from build123d import *

# Parameters (mm, degrees)
F0_W     = 400
F0_H     = 500
F1_DEPTH = 750
F3_DEPTH = 20
F4_W     = 380
F4_H     = 480
F5_DEPTH = 618.889272


with BuildPart() as f1:
    # F0 (on Front) → F1 (new body)
    with BuildSketch(Plane.XZ):
        with Locations((200, 250)):
            Rectangle(F0_W, F0_H)
    extrude(amount=F1_DEPTH)

    # F2 (on face) → F3 (cut)
    with BuildSketch(Plane.XZ.offset(750)):
        Polygon((50, 70), (56, 70), (344, 430), (50, 430), align=None)
        Polygon((344, 430), (56, 70), (350, 70), (350, 430), align=None)
    extrude(amount=-F3_DEPTH, mode=Mode.SUBTRACT)

    # F4 (on face) → F5 (cut)
    with BuildSketch(Plane.XZ.offset(730)):
        with Locations((200, 250)):
            Rectangle(F4_W, F4_H)
    extrude(amount=-F5_DEPTH, mode=Mode.SUBTRACT)


solid = f1.part
Verification items for the finished model (mm, model axes). A direction names the side the tool comes from. Give positions to 0.01 mm unless a question says otherwise; leave off trailing zeros. Write each loop counter-clockwise with the first axis right and the second up, starting at its lowest first coordinate (ties: lowest second). Pieces come first, ordered by that corner, then holes. Notation, with made-up numbers: (83.25, 40) -> (101.25, 40) arc R16 ccw to (101.25, 69) -> close; hole circle Ø4 at (59.25, -18). An arc over 180 degrees is marked (long way). Use CSV: the item, a comma, the result in double quotes.
(1) Set-up check for faces 5 (the flat face through (350, -740, 247)), 6 (the flat face through (390, -425, 247)), 7 (the flat face through (400, -370, 247)): record each of +Z, -Z, +X, -X, +Y, -Y from which the full face is reachable in a straight line by a thin tool's end or side.
Derived:
face 5,"-Y"
face 6,"none"
face 7,"+Z, -Z, +X, +Y, -Y"
(2) Sectioned sample at A-A (x = 362). Record the cut outline in (y, z).
Derived:
outline,"(-750, 0) -> (0, 0) -> (0, 500) -> (-750, 500) -> close; hole (-730, 10) -> (-111.11, 10) -> (-111.11, 490) -> (-730, 490) -> close"
(3) Release check for a two-part mould opening along Y. For faces 1 (the flat face through (10, -425, 247)), 2 (the flat face through (197, 0, 254)), 3 (the flat face through (202, -740, 430)), 4 (the flat face through (375, -750, 254)) record: +Y half, -Y half, draft (parallel to the pull), parting line (faces both ways), or undercut.
Derived:
face 1,"undercut"
face 2,"+Y half"
face 3,"draft"
face 4,"-Y half"
(4) Material ranges on L1, parallel to Y at x = 20, z = 186; L2, parallel to Z at x = 285.5, y = -137.5; L3, parallel to X at y = -637.5, z = 77, recorded low to high.
Derived:
L1,"y = -750 to -730, -111.11 to 0"
L2,"z = 0 to 10, 490 to 500"
L3,"x = 0 to 10, 390 to 400"
(5) Sectioned sample at D-D (x = 148.5). Record the cut outline in (y, z).
Derived:
outline,"(-750, 0) -> (0, 0) -> (0, 500) -> (-750, 500) -> (-750, 430) -> (-730, 430) -> (-730, 490) -> (-111.11, 490) -> (-111.11, 10) -> (-730, 10) -> (-730, 70) -> (-750, 70) -> close"
(6) Sectioned sample at C-C (z = 197.5). Record the cut outline in (x, y), plus the area to 3 significant figures.
Derived:
outline,"(0, -750) -> (50, -750) -> (50, -730) -> (10, -730) -> (10, -111.11) -> (390, -111.11) -> (390, -730) -> (350, -730) -> (350, -750) -> (400, -750) -> (400, 0) -> (0, 0) -> close"
area,"58,800 mm^2"
(7) Sectioned sample at B-B (y = -547). Record the cut outline in (x, z), plus the area to 3 significant figures.
Derived:
outline,"(0, 0) -> (400, 0) -> (400, 500) -> (0, 500) -> close; hole (10, 10) -> (390, 10) -> (390, 490) -> (10, 490) -> close"
area,"17,600 mm^2"
(8) Go/stop test with a flat-tipped pin: pin 1 (2 mm diameter, centred on x = 253, z = 331.5, fed in from -Y). Record where the tip stops, or that it passes through.
Derived:
pin 1,"stops at y = -111.11"
